from build123d import *

# Parameters (mm, degrees)
BOSS_EXTRUDE1_DEPTH        = 38.1
F_1_2_0_5_DIAMETER_HOLE1_D = 12.7
SKETCH4_R                  = 22.225
CUT_EXTRUDE1_DEPTH         = 104.953980203
F_3_8_24_TAPPED_HOLE1_D    = 8.4328


with BuildPart() as part:
    # Sketch1 → Boss-Extrude1 (new, symmetric)
    with BuildSketch(Plane.XY):
        with BuildLine():
            Line((-88.9, 31.75), (-88.9, -6.35))
            Line((-88.9, -6.35), (71.755, -6.35))
            ThreePointArc((71.755, -6.35), (74.898089642, -7.651910358), (76.2, -10.795))
            Line((76.2, -10.795), (76.2, -31.75))
            Line((76.2, -31.75), (88.9, -31.75))
            Line((88.9, -31.75), (88.9, 6.35))
            Line((88.9, 6.35), (-71.755, 6.35))
            ThreePointArc((-71.755, 6.35), (-74.898089642, 7.651910358), (-76.2, 10.795))
            Line((-76.2, 10.795), (-76.2, 31.75))
            Line((-76.2, 31.75), (-88.9, 31.75))
        make_face()
    extrude(amount=BOSS_EXTRUDE1_DEPTH, both=True)

    # 1/2 (0.5) Diameter Hole1 (through all)
    with Locations(Plane(origin=(88.9, 0, 0), x_dir=(0, 0, -1), z_dir=(1, 0, 0))):
        with Locations((-23.606482726, -19.05), (14.493517274, -19.05), (-23.606482726, 19.05), (14.493517274, 19.05)):
            Hole(F_1_2_0_5_DIAMETER_HOLE1_D / 2)

    # Sketch4 → Cut-Extrude1 (cut, through all)
    with BuildSketch(Plane(origin=(0, 6.35, 0), x_dir=(1, 0, 0), z_dir=(0, 1, 0))):
        with Locations(Location((0, 0, 0), (0, 0, 180))):
            Circle(SKETCH4_R)
    extrude(amount=-CUT_EXTRUDE1_DEPTH, mode=Mode.SUBTRACT)

    # 3/8-24 Tapped Hole1 (through all)
    with Locations(Plane(origin=(0, 6.35, 0), x_dir=(1, 0, 0), z_dir=(0, 1, 0))):
        with Locations((44.45, 0), (-44.45, 0)):
            Hole(F_3_8_24_TAPPED_HOLE1_D / 2)


solid = part.part
Read the model definition and answer for the solid it produces. Units are mm, in the model's axes. A direction names the side the tool comes from. Give positions to 0.01 mm unless a question says otherwise; leave off trailing zeros. Loops run counter-clockwise (first coordinate to the right, second up) from the corner with the lowest first, then second, coordinate; pieces in that order, holes last. Notation, with made-up numbers: (86.25, -34) - (105.25, -34) arc R18 cw to (105.25, -26) - close; hole circle Ø11 at (-6.5, 87). An arc over 180 degrees is marked (long way). Answer as CSV lines item,"result". Start each with the question number.
1) Straight lines are drawn through the part: L1, parallel to Z at x = 80, y = -19; L2, parallel to Z at x = 0, y = 2 (3 decimals); L3, parallel to Z at x = 44.45, y = 0. For each, find the intervals that lie inside material, in ascending order. Write a range as from..to.
2) Find section A-A (z = 0). Write down the section's boundary in (x, y) (3 decimals).
3) Find section C-C (y = 0). Write down the section's boundary in (x, z) (3 decimals).
4) Determine the mould class of faces 1 (the face through (-74.863, 7.618, 0.533)), 2 (the face through (16.4, 0.1, 15)), 3 (the face through (82.461, -21.482, -8.628)) for opening direction X: released by +X, released by -X, zero draft, split by the parting line, or undercut.
5) Find section D-D (y = 19.05). Write down the section's boundary in (x, z), then the cut area to 3 significant figures.
6) Each of these flat-tipped pins is pushed along its axis until it touches: pin 1 Ø6.5 at (y, z) = (26.5, -3.5) entering from +X; pin 2 Ø9.5 at (x, z) = (44.45, 0) entering from +Y; pin 3 Ø10.5 at (y, z) = (-26, -9) entering from -X; pin 4 Ø10 at (y, z) = (19.05, 23.61) entering from -X. Where does it stop, or does it pass through?
7) Which of the six approach directions +Z, -Z, +X, -X, +Y, -Y give full straight-line access (tool end or side, diameter ignored) to faces 4 (the face through (48.662, -0.089, -0.185)), 5 (the face through (76.2, -21, 1)), 6 (the face through (-76.2, 21, 1))?
8) Find section B-B (x = 0). Write down the section's boundary in (y, z) (3 decimals).
Findings below:
1,L1,"-38.1..-20.84, -8.14..17.26, 29.96..38.1"
1,L2,"-38.1..-22.225, 22.225..38.1"
1,L3,"-38.1..-4.22, 4.22..38.1"
2,outline,"(-88.9, -6.35) - (-48.666, -6.35) - (-48.666, 6.35) - (-71.755, 6.35) arc R4.445 cw to (-76.2, 10.795) - (-76.2, 31.75) - (-88.9, 31.75) - close; (-40.234, -6.35) - (-22.225, -6.35) - (-22.225, 6.35) - (-40.234, 6.35) - close; (22.225, -6.35) - (40.234, -6.35) - (40.234, 6.35) - (22.225, 6.35) - close; (48.666, -6.35) - (71.755, -6.35) arc R4.445 cw to (76.2, -10.795) - (76.2, -31.75) - (88.9, -31.75) - (88.9, 6.35) - (48.666, 6.35) - close"
3,outline,"(-88.9, -38.1) - (88.9, -38.1) - (88.9, 38.1) - (-88.9, 38.1) - close; hole circle Ø8.433 at (-44.45, 0); hole circle Ø44.45 at (0, 0); hole circle Ø8.433 at (44.45, 0)"
4,face 1,"released by +X"
4,face 2,"undercut"
4,face 3,"zero draft"
5,outline,"(-88.9, -38.1) - (-76.2, -38.1) - (-76.2, -20.84) - (-88.9, -20.84) - close; (-88.9, -8.14) - (-76.2, -8.14) - (-76.2, 17.26) - (-88.9, 17.26) - close; (-88.9, 29.96) - (-76.2, 29.96) - (-76.2, 38.1) - (-88.9, 38.1) - close"
5,area,"645 mm^2"
6,pin 1,"x = -76.2"
6,pin 2,"y = 6.35"
6,pin 3,"x = 76.2"
6,pin 4,"through"
7,face 4,"+Y, -Y"
7,face 5,"+Z, -Z, -X, -Y"
7,face 6,"+Z, -Z, +X, +Y"
8,outline,"(-6.35, -38.1) - (6.35, -38.1) - (6.35, -22.225) - (-6.35, -22.225) - close; (-6.35, 22.225) - (6.35, 22.225) - (6.35, 38.1) - (-6.35, 38.1) - close"
